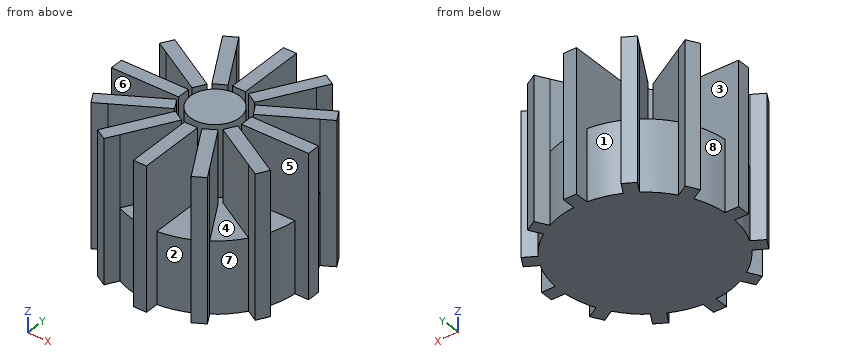
```python
from build123d import *

# Parameters (mm, degrees)
F0_R     = 8.734171
F1_DEPTH = 25
F2_DEPTH = 50


with BuildPart() as f1:
    # F0 (on Top) → F1 (new body)
    with BuildSketch(Plane.XY):
        with BuildLine():
            Line((11.107184, 2.346986), (29.908053, 2.346986))
            ThreePointArc((29.908053, 2.346986), (28.967814, 7.801649), (27.041466, 12.990731))
            Line((27.041466, 12.990731), (10.754318, 3.587342))
            Line((10.754318, 3.587342), (8.44561, 7.586142))
            Line((8.44561, 7.586142), (24.727641, 16.986576))
            ThreePointArc((24.727641, 16.986576), (21.186039, 21.240333), (16.923231, 24.771036))
            Line((16.923231, 24.771036), (7.519842, 8.483889))
            Line((7.519842, 8.483889), (3.521042, 10.792597))
            Line((3.521042, 10.792597), (12.921477, 27.074627))
            ThreePointArc((12.921477, 27.074627), (7.727481, 28.987688), (2.27043, 29.913962))
            Line((2.27043, 29.913962), (2.27043, 11.107184))
            Line((2.27043, 11.107184), (-2.346986, 11.107184))
            Line((-2.346986, 11.107184), (-2.346986, 29.908053))
            ThreePointArc((-2.346986, 29.908053), (-7.801649, 28.967814), (-12.990731, 27.041466))
            Line((-12.990731, 27.041466), (-3.587342, 10.754318))
            Line((-3.587342, 10.754318), (-7.586142, 8.44561))
            Line((-7.586142, 8.44561), (-16.986576, 24.727641))
            ThreePointArc((-16.986576, 24.727641), (-21.240333, 21.186039), (-24.771036, 16.923231))
            Line((-24.771036, 16.923231), (-8.483889, 7.519842))
            Line((-8.483889, 7.519842), (-10.792597, 3.521042))
            Line((-10.792597, 3.521042), (-27.074627, 12.921477))
            ThreePointArc((-27.074627, 12.921477), (-28.987688, 7.727481), (-29.913962, 2.27043))
            Line((-29.913962, 2.27043), (-11.107184, 2.27043))
            Line((-11.107184, 2.27043), (-11.107184, -2.346986))
            Line((-11.107184, -2.346986), (-29.908053, -2.346986))
            ThreePointArc((-29.908053, -2.346986), (-28.967814, -7.801649), (-27.041466, -12.990731))
            Line((-27.041466, -12.990731), (-10.754318, -3.587342))
            Line((-10.754318, -3.587342), (-8.44561, -7.586142))
            Line((-8.44561, -7.586142), (-24.727641, -16.986576))
            ThreePointArc((-24.727641, -16.986576), (-21.186039, -21.240333), (-16.923231, -24.771036))
            Line((-16.923231, -24.771036), (-7.519842, -8.483889))
            Line((-7.519842, -8.483889), (-3.521042, -10.792597))
            Line((-3.521042, -10.792597), (-12.921477, -27.074627))
            ThreePointArc((-12.921477, -27.074627), (-7.727481, -28.987688), (-2.27043, -29.913962))
            Line((-2.27043, -29.913962), (-2.27043, -11.107184))
            Line((-2.27043, -11.107184), (2.346986, -11.107184))
            Line((2.346986, -11.107184), (2.346986, -29.908053))
            ThreePointArc((2.346986, -29.908053), (7.801649, -28.967814), (12.990731, -27.041466))
            Line((12.990731, -27.041466), (3.587342, -10.754318))
            Line((3.587342, -10.754318), (7.586142, -8.44561))
            Line((7.586142, -8.44561), (16.986576, -24.727641))
            ThreePointArc((16.986576, -24.727641), (21.240333, -21.186039), (24.771036, -16.923231))
            Line((24.771036, -16.923231), (8.483889, -7.519842))
            Line((8.483889, -7.519842), (10.792597, -3.521042))
            Line((10.792597, -3.521042), (27.074627, -12.921477))
            ThreePointArc((27.074627, -12.921477), (28.987688, -7.727481), (29.913962, -2.27043))
            Line((29.913962, -2.27043), (11.107184, -2.27043))
            Line((11.107184, -2.27043), (11.107184, 2.346986))
        make_face()
        Circle(F0_R, mode=Mode.SUBTRACT)
    extrude(amount=F1_DEPTH)

    # F0 (on Top) → F2 (join)
    with BuildSketch(Plane.XY):
        with BuildLine():
            ThreePointArc((-27.074627, 12.921477), (-25.999937, 14.966739), (-24.771036, 16.923231))
            Line((-24.771036, 16.923231), (-28.949671, 19.335767))
            Line((-28.949671, 19.335767), (-31.258379, 15.336967))
            Line((-31.258379, 15.336967), (-27.074627, 12.921477))
        make_face()
        with BuildLine():
            ThreePointArc((-16.986576, 24.727641), (-15.033236, 25.961545), (-12.990731, 27.041466))
            Line((-12.990731, 27.041466), (-15.403267, 31.220101))
            Line((-15.403267, 31.220101), (-19.402067, 28.911393))
            Line((-19.402067, 28.911393), (-16.986576, 24.727641))
        make_face()
        with BuildLine():
            ThreePointArc((-2.346986, 29.908053), (-0.038392, 29.999975), (2.27043, 29.913962))
            Line((2.27043, 29.913962), (2.27043, 34.739034))
            Line((2.27043, 34.739034), (-2.346986, 34.739034))
            Line((-2.346986, 34.739034), (-2.346986, 29.908053))
        make_face()
        with BuildLine():
            ThreePointArc((12.921477, 27.074627), (14.966739, 25.999937), (16.923231, 24.771036))
            Line((16.923231, 24.771036), (19.335767, 28.949671))
            Line((19.335767, 28.949671), (15.336967, 31.258379))
            Line((15.336967, 31.258379), (12.921477, 27.074627))
        make_face()
        with BuildLine():
            ThreePointArc((24.727641, 16.986576), (25.961545, 15.033236), (27.041466, 12.990731))
            Line((27.041466, 12.990731), (31.220101, 15.403267))
            Line((31.220101, 15.403267), (28.911393, 19.402067))
            Line((28.911393, 19.402067), (24.727641, 16.986576))
        make_face()
        with BuildLine():
            ThreePointArc((29.908053, 2.346986), (29.977005, 1.174393), (30, 0))
            ThreePointArc((30, 0), (29.978483, -1.13603), (29.913962, -2.27043))
            Line((29.913962, -2.27043), (34.739034, -2.27043))
            Line((34.739034, -2.27043), (34.739034, 2.346986))
            Line((34.739034, 2.346986), (29.908053, 2.346986))
        make_face()
        with BuildLine():
            Line((31.258379, -15.336967), (27.074627, -12.921477))
            ThreePointArc((27.074627, -12.921477), (25.999937, -14.966739), (24.771036, -16.923231))
            Line((24.771036, -16.923231), (28.949671, -19.335767))
            Line((28.949671, -19.335767), (31.258379, -15.336967))
        make_face()
        with BuildLine():
            Line((19.402067, -28.911393), (16.986576, -24.727641))
            ThreePointArc((16.986576, -24.727641), (15.033236, -25.961545), (12.990731, -27.041466))
            Line((12.990731, -27.041466), (15.403267, -31.220101))
            Line((15.403267, -31.220101), (19.402067, -28.911393))
        make_face()
        with BuildLine():
            ThreePointArc((12.990731, -27.041466), (15.033236, -25.961545), (16.986576, -24.727641))
            Line((16.986576, -24.727641), (7.586142, -8.44561))
            Line((7.586142, -8.44561), (3.587342, -10.754318))
            Line((3.587342, -10.754318), (12.990731, -27.041466))
        make_face()
        with BuildLine():
            ThreePointArc((24.771036, -16.923231), (25.999937, -14.966739), (27.074627, -12.921477))
            Line((27.074627, -12.921477), (10.792597, -3.521042))
            Line((10.792597, -3.521042), (8.483889, -7.519842))
            Line((8.483889, -7.519842), (24.771036, -16.923231))
        make_face()
        with BuildLine():
            ThreePointArc((29.913962, -2.27043), (29.978483, -1.13603), (30, 0))
            ThreePointArc((30, 0), (29.977005, 1.174393), (29.908053, 2.346986))
            Line((29.908053, 2.346986), (11.107184, 2.346986))
            Line((11.107184, 2.346986), (11.107184, -2.27043))
            Line((11.107184, -2.27043), (29.913962, -2.27043))
        make_face()
        with BuildLine():
            Line((10.754318, 3.587342), (27.041466, 12.990731))
            ThreePointArc((27.041466, 12.990731), (25.961545, 15.033236), (24.727641, 16.986576))
            Line((24.727641, 16.986576), (8.44561, 7.586142))
            Line((8.44561, 7.586142), (10.754318, 3.587342))
        make_face()
        with BuildLine():
            Line((7.519842, 8.483889), (16.923231, 24.771036))
            ThreePointArc((16.923231, 24.771036), (14.966739, 25.999937), (12.921477, 27.074627))
            Line((12.921477, 27.074627), (3.521042, 10.792597))
            Line((3.521042, 10.792597), (7.519842, 8.483889))
        make_face()
        with BuildLine():
            Line((2.27043, 11.107184), (2.27043, 29.913962))
            ThreePointArc((2.27043, 29.913962), (-0.038392, 29.999975), (-2.346986, 29.908053))
            Line((-2.346986, 29.908053), (-2.346986, 11.107184))
            Line((-2.346986, 11.107184), (2.27043, 11.107184))
        make_face()
        with BuildLine():
            Line((-3.587342, 10.754318), (-12.990731, 27.041466))
            ThreePointArc((-12.990731, 27.041466), (-15.033236, 25.961545), (-16.986576, 24.727641))
            Line((-16.986576, 24.727641), (-7.586142, 8.44561))
            Line((-7.586142, 8.44561), (-3.587342, 10.754318))
        make_face()
        with BuildLine():
            Line((-8.483889, 7.519842), (-24.771036, 16.923231))
            ThreePointArc((-24.771036, 16.923231), (-25.999937, 14.966739), (-27.074627, 12.921477))
            Line((-27.074627, 12.921477), (-10.792597, 3.521042))
            Line((-10.792597, 3.521042), (-8.483889, 7.519842))
        make_face()
        with BuildLine():
            ThreePointArc((-29.908053, -2.346986), (-29.999975, -0.038392), (-29.913962, 2.27043))
            Line((-29.913962, 2.27043), (-34.739034, 2.27043))
            Line((-34.739034, 2.27043), (-34.739034, -2.346986))
            Line((-34.739034, -2.346986), (-29.908053, -2.346986))
        make_face()
        with BuildLine():
            Line((-28.911393, -19.402067), (-24.727641, -16.986576))
            ThreePointArc((-24.727641, -16.986576), (-25.961545, -15.033236), (-27.041466, -12.990731))
            Line((-27.041466, -12.990731), (-31.220101, -15.403267))
            Line((-31.220101, -15.403267), (-28.911393, -19.402067))
        make_face()
        with BuildLine():
            ThreePointArc((-27.041466, -12.990731), (-25.961545, -15.033236), (-24.727641, -16.986576))
            Line((-24.727641, -16.986576), (-8.44561, -7.586142))
            Line((-8.44561, -7.586142), (-10.754318, -3.587342))
            Line((-10.754318, -3.587342), (-27.041466, -12.990731))
        make_face()
        with BuildLine():
            ThreePointArc((-16.923231, -24.771036), (-14.966739, -25.999937), (-12.921477, -27.074627))
            Line((-12.921477, -27.074627), (-3.521042, -10.792597))
            Line((-3.521042, -10.792597), (-7.519842, -8.483889))
            Line((-7.519842, -8.483889), (-16.923231, -24.771036))
        make_face()
        with BuildLine():
            Line((-15.336967, -31.258379), (-12.921477, -27.074627))
            ThreePointArc((-12.921477, -27.074627), (-14.966739, -25.999937), (-16.923231, -24.771036))
            Line((-16.923231, -24.771036), (-19.335767, -28.949671))
            Line((-19.335767, -28.949671), (-15.336967, -31.258379))
        make_face()
        with BuildLine():
            ThreePointArc((-2.27043, -29.913962), (0.038392, -29.999975), (2.346986, -29.908053))
            Line((2.346986, -29.908053), (2.346986, -11.107184))
            Line((2.346986, -11.107184), (-2.27043, -11.107184))
            Line((-2.27043, -11.107184), (-2.27043, -29.913962))
        make_face()
        with BuildLine():
            Line((2.346986, -34.739034), (2.346986, -29.908053))
            ThreePointArc((2.346986, -29.908053), (0.038392, -29.999975), (-2.27043, -29.913962))
            Line((-2.27043, -29.913962), (-2.27043, -34.739034))
            Line((-2.27043, -34.739034), (2.346986, -34.739034))
        make_face()
        Circle(F0_R)
        with BuildLine():
            Line((-11.107184, 2.27043), (-29.913962, 2.27043))
            ThreePointArc((-29.913962, 2.27043), (-29.999975, -0.038392), (-29.908053, -2.346986))
            Line((-29.908053, -2.346986), (-11.107184, -2.346986))
            Line((-11.107184, -2.346986), (-11.107184, 2.27043))
        make_face()
    extrude(amount=F2_DEPTH)


solid = f1.part
```
The model under review builds one solid part; all positions refer to its coordinate system, in mm. Face numbers are marked on the shaded views. A direction names the side the tool comes from. Round coordinates to 2 decimals unless told otherwise and drop trailing zeros. Loops run counter-clockwise (first coordinate to the right, second up) from the corner with the lowest first, then second, coordinate; pieces in that order, holes last. Notation, with made-up numbers: (1, 23) -> (22, 23) arc R21 ccw to (22, 43) -> close; hole circle Ø8 at (-0.5, 79.25). An arc over 180 degrees is marked (long way). Answer in a Markdown table with one row per item.
1) Tool access review of the marked faces 5, 6, 7 and 8: name each direction out of +Z, -Z, +X, -X, +Y, -Y from which nothing blocks a thin tool from reaching the whole face with its end or side.
Taken from the geometry:
| item | result |
|---|---|
| face 5 | +Z, +X |
| face 6 | +Z, -X |
| face 7 | +Z, -Z |
| face 8 | +Z, -Z, -X |
2) Wall thickness on line 1 along X through (y, z) = (0.5, 42); line 2 along Y through (x, z) = (-21, 30.5); line 3 along Y through (x, z) = (-9, 45): over which ranges is each line inside the solid? List them lowest first.
Taken from the geometry:
| item | result |
|---|---|
| line 1 | x = -34.74 to -11.11, -8.72 to 8.72, 11.11 to 34.74 |
| line 2 | y = -14.83 to -9.5, -2.35 to 2.27, 9.41 to 14.75 |
| line 3 | y = -20.28 to -11.05, -7.91 to -6.63, 6.63 to 7.82, 10.89 to 20.13 |
3) Consider section A-A, the plane z = 29.5. Count the separate pieces of the cut face and the enclosed holes in it, plus the area to 3 significant figures.
Taken from the geometry:
| item | result |
|---|---|
| separate pieces | 13 |
| enclosed holes | 0 |
| area | 1,550 mm² |
4) Consider section B-B, the plane x = 0. Write out the cut boundary in (y, z).
Taken from the geometry:
| item | result |
|---|---|
| outline | (-34.74, 0) -> (34.74, 0) -> (34.74, 50) -> (11.11, 50) -> (11.11, 25) -> (8.73, 25) -> (8.73, 50) -> (-8.73, 50) -> (-8.73, 25) -> (-11.11, 25) -> (-11.11, 50) -> (-34.74, 50) -> close |
5) For pin 1 Ø1.5 at (y, z) = (-20.5, 28.5) entering from +X; pin 2 Ø12 at (y, z) = (28, 29.5) entering from -X; pin 3 Ø5 at (y, z) = (-4.5, 13) entering from -X; pin 4 Ø2 at (y, z) = (20, 9) entering from +X, all flat-tipped, find the tip position at first contact; note any pin that passes through.
Taken from the geometry:
| item | result |
|---|---|
| pin 1 | stops at x = 14.98 |
| pin 2 | stops at x = -19.4 |
| pin 3 | stops at x = -34.74 |
| pin 4 | stops at x = 29.14 |
6) Draft analysis for pull direction Y (two halves, no side actions). For the marked faces 1, 2, 3 and 4, state which applies: pulls with the +Y half, pulls with the -Y half, needs draft (parallel to the pull), parting line crosses it, or undercut.
Taken from the geometry:
| item | result |
|---|---|
| face 1 | pulls with the +Y half |
| face 2 | pulls with the -Y half |
| face 3 | undercut |
| face 4 | undercut |
